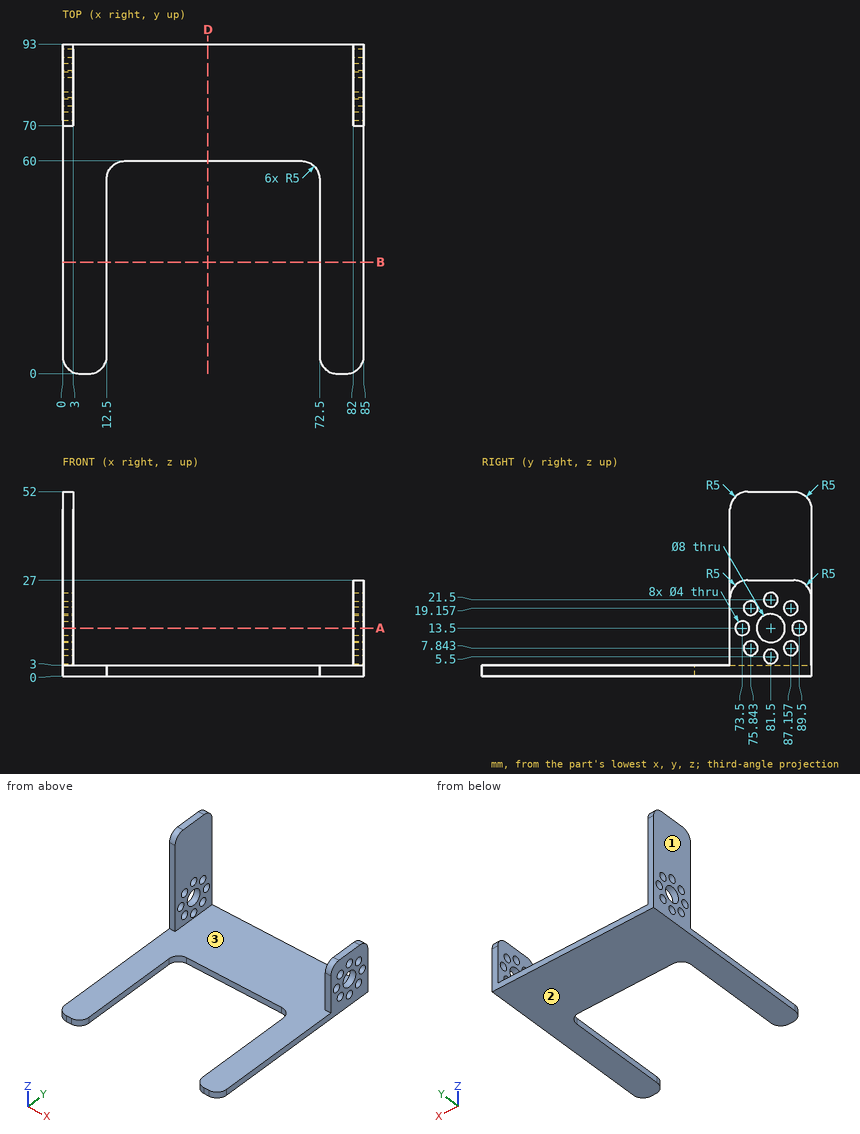
Answer from the drawing. Dimensions are ordinates in mm from the lowest x, y and z of the part. Give positions to 0.01 mm unless a question says otherwise; leave off trailing zeros. Loops run counter-clockwise (first coordinate to the right, second up) from the corner with the lowest first, then second, coordinate; pieces in that order, holes last. Notation, with made-up numbers: (-38, 80.5) - (0, 80.5) arc R17 ccw to (0, 95.5) - close; hole circle Ø7 at (69, -14). An arc over 180 degrees is marked (long way). Write each question's results on one line, items separated by ' | '.
1. Find section B-B, the plane y = 31.5. Write down the section's boundary in (x, z), then the cut area to 3 significant figures.
Resolved:
outline: (0, 0) - (12.5, 0) - (12.5, 3) - (0, 3) - close; (72.5, 0) - (85, 0) - (85, 3) - (72.5, 3) - close | area: 75.0 mm^2
2. Consider probe 1 along Y at (x, z) = (83, 13); probe 2 along Z at (x, y) = (18, 67.5). Determine where each line is inside the solid, lowest interval first. Write a range as from..to.
Resolved:
probe 1: y = 70..71.56, 75.44..77.53, 85.47..87.56, 91.44..93 | probe 2: z = 0..3
3. Flat-ended cylindrical pins translate along their axes: P1, Ø1.5, axis at x = 83, z = 10, coming from the -Y side; P2, Ø5, axis at x = 65.5, z = 6, coming from the +Y side; P3, Ø1.5, axis at x = 83, y = 80, coming from the +Z side; P4, Ø1.5, axis at x = 34.5, z = 1.5, coming from the -Y side. Find the tip coordinate at first contact, or state that the pin passes through.
Resolved:
P1: stops at y = 70 | P2: passes through | P3: stops at z = 27 | P4: stops at y = 60
4. Find section D-D, the plane x = 41. Write down the section's boundary in (y, z), then the cut area to 3 significant figures.
Resolved:
outline: (60, 0) - (93, 0) - (93, 3) - (60, 3) - close | area: 99.0 mm^2
5. For a pull along X with two mould halves and no side action, classify the marked faces 1, 2 and 3 as +X half, -X half, draft (parallel to the pull), parting line (faces both ways), or undercut.
Resolved:
face 1: -X half | face 2: draft | face 3: undercut
6. Find section A-A, the plane z = 13.5. Count the separate pieces of the cut face and the enclosed holes in it, then the cut area to 3 significant figures.
Resolved:
separate pieces: 8 | enclosed holes: 0 | area: 42.0 mm^2
